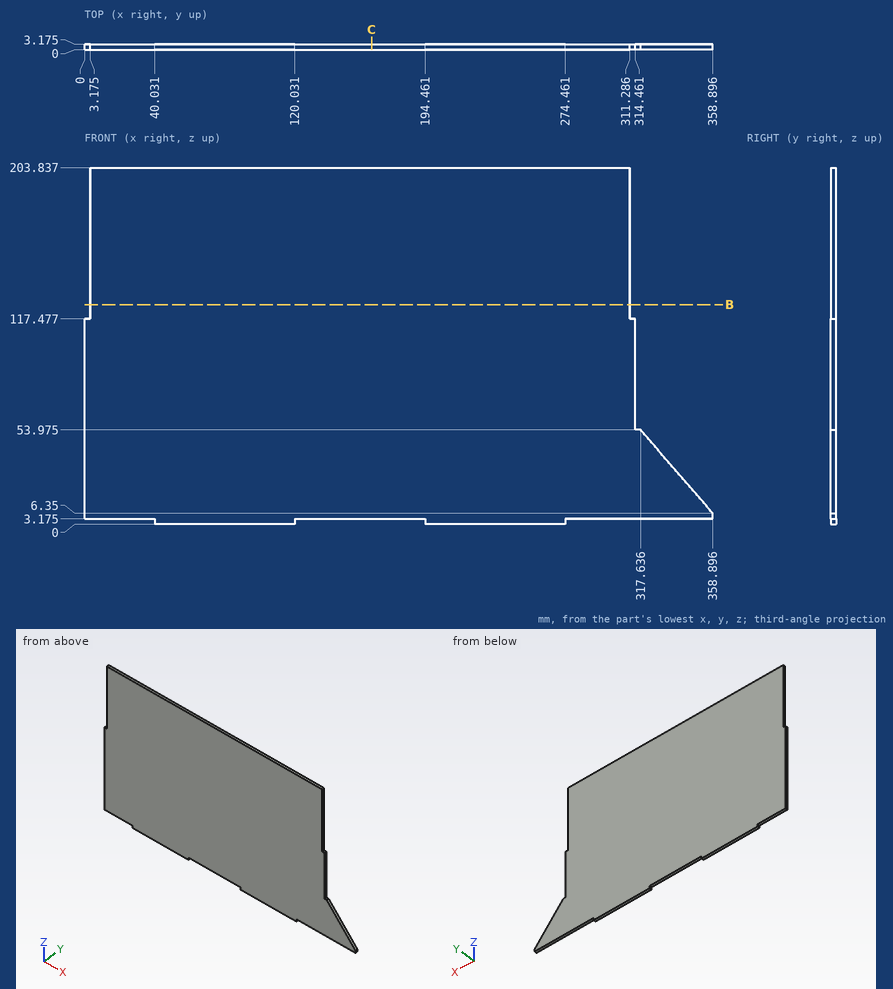
Answer from the drawing. Dimensions are ordinates in mm from the lowest x, y and z of the part. Give positions to 0.01 mm unless a question says otherwise; leave off trailing zeros. Order: outer loops, then holes, each group sorted by start corner. A loop starts at its lowest first (then second) coordinate and runs counter-clockwise, first axis right, second up. Notation, with made-up numbers: (-2, 69) -> (47, 69) arc R13 cw to (47, 80) -> close; hole circle Ø1 at (43.25, 45.5). An arc over 180 degrees is marked (long way). Answer as a JSON object with one key per item and string values. Group by question number.
1. Consider line 1 along X through (y, z) = (2.9, 139.5) (1 decimal); line 2 along X through (y, z) = (1.6, 82.5); line 3 along Z through (x, y) = (126.5, 0.65) (1 decimal). Determine where each line is inside the solid, lowest interval first. Write a range as [from, to].
2. Section C-C on x = 164 is taken. Determine the outline of the cut face in (y, z) (1 decimal), plus the area to 3 significant figures.
3. Section B-B on z = 125.5 is taken. Determine the outline of the cut face in (x, y) (1 decimal).
4. Flat-ended cylindrical pins translate along their axes: pin 1 Ø1.6 at (y, z) = (1.5, 2) entering from -X; pin 2 Ø1.6 at (y, z) = (2, 180) entering from +X; pin 3 Ø1 at (y, z) = (1.5, 182) entering from -X (3 decimals). Find the tip coordinate at first contact, or state that the pin passes through.
Result sheet:
{
 "1": {"line 1": "x = [3.2, 311.3]", "line 2": "x = [0, 314.46]", "line 3": "z = [3.2, 203.8]"},
 "2": {"outline": "(0, 3.2) -> (3.2, 3.2) -> (3.2, 203.8) -> (0, 203.8) -> close", "area": "637 mm^2"},
 "3": {"outline": "(3.2, 0) -> (311.3, 0) -> (311.3, 3.2) -> (3.2, 3.2) -> close"},
 "4": {"pin 1": "stops at x = 40.03", "pin 2": "stops at x = 311.29", "pin 3": "stops at x = 3.175"}
}
